Check sheet for the modelled part. Datum: model origin and axes. Units: mm. A direction names the side the tool comes from. Round coordinates to 2 decimals unless told otherwise and drop trailing zeros. Order: outer loops, then holes, each group sorted by start corner. A loop starts at its lowest first (then second) coordinate and runs counter-clockwise, first axis right, second up. Notation, with made-up numbers: (-31.75, 74.25) -> (-2.75, 74.25) arc R20 cw to (-2.75, 101.25) -> close; hole circle Ø4 at (59.5, 50.25). An arc over 180 degrees is marked (long way). Answer in a Markdown table with one row per item. Add a question column.
1. Depth check by flat-ended pin: P1, Ø0.8, axis at y = 69.5, z = 1, coming from the -X side; P2, Ø0.8, axis at x = 64, z = 1, coming from the -Y side (3 decimals); P3, Ø0.8, axis at x = 63, z = 0.5, coming from the +Y side. Enter the tip coordinate at first touch or a pass-through.
2. Access from +Z, -Z, +X, -X, +Y, -Y to the whole of each face (thin tool, end or side, straight path). Record for faces 4 (the cylindrical face through (155.926, 37.035, 0.751)), 5 (the flat face through (94, 67, 1.524)), 6 (the cylindrical face through (98.676, 42.006, 0.751)), 7 (the flat face through (75.21, 80.36, 0.75)), 8 (the cylindrical face through (46.88, 116.58, 0.75)).
3. Draft check along X on faces 1 (the flat face through (53.76, 125.37, 0.75)), 2 (the cylindrical face through (120.64, 63.54, 0.75)), 3 (the cylindrical face through (122.99, 37.86, 0.75)). Enter one of: +X half, -X half, draft (parallel to the pull), parting line (faces both ways), or undercut.
4. Sectioned sample at B-B, the plane y = 53. Record the boundary of the cut face in (x, z).
5. Sectioned sample at A-A, the plane x = 87. Record the boundary of the cut face in (y, z), then the cut area to 3 significant figures.
6. Material ranges on L1, parallel to X at y = 103, z = 0.55; L2, parallel to X at y = 104, z = 1; L3, parallel to X at y = 42, z = 0.6, recorded low to high. Write a range as from..to.
7. Sectioned sample at C-C, the plane x = 127. Record the boundary of the cut face in (y, z), then the cut area to 3 significant figures.
```python
from build123d import *

# Parameters (mm, degrees)
BOSS_EXTRUDE1_DEPTH = 1.524


with BuildPart() as part:
    # Sketch1 → Boss-Extrude1 (new body)
    with BuildSketch(Plane.XY):
        with BuildLine():
            Line((56.264141338, 126.956858816), (51.174858052, 123.732229714))
            Line((51.174858052, 123.732229714), (53.307781304, 120.365935384))
            Line((53.307781304, 120.365935384), (52.020439004, 119.550260325))
            Line((52.020439004, 119.550260325), (49.887515751, 122.916554654))
            Line((49.887515751, 122.916554654), (44.798232465, 119.691925553))
            ThreePointArc((44.798232465, 119.691925553), (46.919348528, 116.541161993), (50.056966547, 114.400648613))
            ThreePointArc((50.056966547, 114.400648613), (52.160922541, 111.249416579), (51.38551555, 107.540557165))
            ThreePointArc((51.38551555, 107.540557165), (48.819467631, 103.01456573), (48.033803289, 97.871421561))
            Line((48.033803289, 97.871421561), (53.714736294, 104.703768794))
            Line((53.714736294, 104.703768794), (54.886575206, 103.729412819))
            Line((54.886575206, 103.729412819), (48.256070281, 95.755033975))
            ThreePointArc((48.256070281, 95.755033975), (48.940021774, 93.270180673), (50.056966547, 90.947527029))
            ThreePointArc((50.056966547, 90.947527029), (51.738858239, 87.952338233), (51.38551555, 84.535458878))
            ThreePointArc((51.38551555, 84.535458878), (51.676023362, 83.881512061), (52.003112941, 83.245073819))
            ThreePointArc((52.003112941, 83.245073819), (51.432071992, 81.656527536), (51.174858052, 79.988172643))
            ThreePointArc((51.174858052, 79.988172643), (52.003112941, 81.035329758), (53.307781304, 81.318851624))
            ThreePointArc((53.307781304, 81.318851624), (54.639987623, 79.928222594), (56.168191464, 78.75637969))
            ThreePointArc((56.168191464, 78.75637969), (56.082073865, 77.101010294), (56.669286419, 75.550898847))
            ThreePointArc((56.669286419, 75.550898847), (56.856082806, 76.879297739), (57.74991105, 77.879601482))
            ThreePointArc((57.74991105, 77.879601482), (58.566064016, 77.535130701), (59.404362787, 77.2487377))
            ThreePointArc((59.404362787, 77.2487377), (59.468887944, 75.800864539), (59.621212135, 74.359581247))
            ThreePointArc((59.621212135, 74.359581247), (58.548532564, 73.021617268), (57.74991105, 71.50405582))
            ThreePointArc((57.74991105, 71.50405582), (58.750795137, 72.225661043), (59.934465672, 72.574096285))
            ThreePointArc((59.934465672, 72.574096285), (60.218266334, 71.399198054), (60.56120896, 70.240181651))
            Line((60.56120896, 70.240181651), (68.053425724, 70.240181651))
            Line((68.053425724, 70.240181651), (68.053425724, 68.651586531))
            Line((68.053425724, 68.651586531), (61.138299457, 68.651586531))
            ThreePointArc((61.138299457, 68.651586531), (64.007218606, 63.496556651), (68.053425724, 59.203161944))
            ThreePointArc((68.053425724, 59.203161944), (72.105402023, 56.054971734), (77.236381434, 56.106583856))
            ThreePointArc((77.236381434, 56.106583856), (78.044746131, 53.287579438), (78.998529881, 50.51439788))
            Line((78.998529881, 50.51439788), (90.459222019, 50.51439788))
            Line((90.459222019, 50.51439788), (90.459222019, 48.97144986))
            Line((90.459222019, 48.97144986), (79.600424402, 48.97144986))
            ThreePointArc((79.600424402, 48.97144986), (80.560218525, 46.751381797), (81.614302179, 44.574499941))
            ThreePointArc((81.614302179, 44.574499941), (88.40638605, 40.908931841), (95.623925921, 43.643143066))
            ThreePointArc((95.623925921, 43.643143066), (98.719457239, 41.9837065), (101.887587861, 40.467463703))
            ThreePointArc((101.887587861, 40.467463703), (104.250570747, 41.59409239), (105.879794993, 43.643143066))
            ThreePointArc((105.879794993, 43.643143066), (105.615285106, 41.362757758), (104.568635279, 39.319562522))
            ThreePointArc((104.568635279, 39.319562522), (108.662838982, 37.791938771), (112.83726515, 36.499536179))
            ThreePointArc((112.83726515, 36.499536179), (114.338838664, 39.431267188), (115.158578251, 42.621533122))
            ThreePointArc((115.158578251, 42.621533122), (115.32642817, 39.283498881), (114.23888805, 36.123134554))
            ThreePointArc((114.23888805, 36.123134554), (117.382688145, 35.380759015), (120.554912672, 34.771175532))
            ThreePointArc((120.554912672, 34.771175532), (123.021749605, 37.9129634), (124.572686361, 41.59409239))
            ThreePointArc((124.572686361, 41.59409239), (124.074787113, 37.838934231), (122.294984417, 34.495071372))
            ThreePointArc((122.294984417, 34.495071372), (126.165693737, 34.02629014), (130.055199537, 33.754460929))
            ThreePointArc((130.055199537, 33.754460929), (132.134455488, 36.288278623), (133.465692892, 39.283498881))
            ThreePointArc((133.465692892, 39.283498881), (133.502994203, 36.396459224), (132.511774167, 33.684656833))
            ThreePointArc((132.511774167, 33.684656833), (136.324034113, 33.731918308), (140.129256944, 33.968220541))
            ThreePointArc((140.129256944, 33.968220541), (140.922011669, 36.642526439), (140.979432276, 39.431267188))
            ThreePointArc((140.979432276, 39.431267188), (141.543710337, 36.799823517), (141.584568778, 34.108869018))
            ThreePointArc((141.584568778, 34.108869018), (145.358502787, 34.60468639), (149.103252173, 35.286789609))
            ThreePointArc((149.103252173, 35.286789609), (149.41526381, 37.485880685), (149.103252173, 39.68497176))
            ThreePointArc((149.103252173, 39.68497176), (150.389458807, 37.857811323), (150.933061601, 35.690476839))
            ThreePointArc((150.933061601, 35.690476839), (155.995803512, 37.056053135), (160.953619193, 38.763746888))
            ThreePointArc((160.953619193, 38.763746888), (120.045431958, 63.84340718), (75.776786754, 82.357083072))
            Line((75.776786754, 82.357083072), (78.55577188, 78.549383563))
            Line((78.55577188, 78.549383563), (77.236381434, 77.586448747))
            Line((77.236381434, 77.586448747), (73.124487989, 83.220467621))
            ThreePointArc((73.124487989, 83.220467621), (70.129640963, 85.609264926), (66.488706533, 86.800507029))
            ThreePointArc((66.488706533, 86.800507029), (65.201078968, 87.547474126), (65.008773799, 89.023605324))
            ThreePointArc((65.008773799, 89.023605324), (65.45394794, 99.671148502), (65.008773799, 110.31869168))
            ThreePointArc((65.008773799, 110.31869168), (64.928240982, 110.624021202), (64.844587925, 110.928510639))
            ThreePointArc((64.844587925, 110.928510639), (63.504830628, 110.096374776), (61.945041493, 109.863013337))
            ThreePointArc((61.945041493, 109.863013337), (63.331098083, 110.928510639), (64.429350166, 112.288760519))
            ThreePointArc((64.429350166, 112.288760519), (63.72134744, 114.213049759), (62.887114334, 116.086071934))
            ThreePointArc((62.887114334, 116.086071934), (61.244379947, 115.688493307), (59.559011987, 115.815693414))
            ThreePointArc((59.559011987, 115.815693414), (61.021114976, 116.355052106), (62.272659221, 117.283647794))
            ThreePointArc((62.272659221, 117.283647794), (61.637025251, 118.402299275), (60.955310984, 119.493480899))
            ThreePointArc((60.955310984, 119.493480899), (59.559011987, 118.734336878), (58.039485129, 118.268516457))
            ThreePointArc((58.039485129, 118.268516457), (59.291178035, 119.385811258), (59.960570457, 120.924315918))
            ThreePointArc((59.960570457, 120.924315918), (59.685184939, 121.291735218), (59.404362787, 121.655016161))
            ThreePointArc((59.404362787, 121.655016161), (59.583464699, 123.412306739), (58.847642556, 125.018144041))
            ThreePointArc((58.847642556, 125.018144041), (57.697156367, 126.175748202), (56.264141338, 126.956858816))
        make_face()
    extrude(amount=BOSS_EXTRUDE1_DEPTH)


solid = part.part
```
Answer key:
| question | item | result |
|---|---|---|
| 1 | P1 | stops at x = 68.05 |
| 1 | P2 | stops at y = 62.975 |
| 1 | P3 | stops at y = 116.09 |
| 2 | face 4 | +Z, -Z, +X, -Y |
| 2 | face 5 | +Z, +X, -X, +Y, -Y |
| 2 | face 6 | +Z, -Z, -Y |
| 2 | face 7 | +Z, -Z |
| 2 | face 8 | +Z, -Z, -X |
| 3 | face 1 | -X half |
| 3 | face 2 | +X half |
| 3 | face 3 | undercut |
| 4 | outline | (78.14, 0) -> (139.49, 0) -> (139.49, 1.52) -> (78.14, 1.52) -> close |
| 5 | outline | (41.11, 0) -> (48.97, 0) -> (48.97, 1.52) -> (41.11, 1.52) -> close; (50.51, 0) -> (78.41, 0) -> (78.41, 1.52) -> (50.51, 1.52) -> close |
| 5 | area | 54.5 mm² |
| 6 | L1 | x = 48.81..52.3, 54.28..65.41 |
| 6 | L2 | x = 49.2..53.13, 54.56..65.38 |
| 6 | L3 | x = 84.62..93.43, 98.69..104.71, 105.77..115.06, 115.29..156.4 |
| 7 | outline | (33.95, 0) -> (60.17, 0) -> (60.17, 1.52) -> (33.95, 1.52) -> close |
| 7 | area | 40.0 mm² |
